Autodesk Inventor part; units mm, degrees
ref_plane "YZ Plane" through (0, 0, 0) normal (1, 0, 0) x (0, 1, 0)
ref_plane "XZ Plane" through (0, 0, 0) normal (0, 1, 0) x (-1, 0, 0)
ref_plane "XY Plane" through (0, 0, 0) normal (0, 0, 1) x (1, 0, 0)
sketch "Sketch1" plane through (0, 0, 0) normal (1, 0, 0) x (0, 1, 0)
  circle A0 centre (0, 0) radius 57.5
  line L0 (0, 0) -> (22.0043, 53.1231)
  line L1 (0, 0) -> (22.0043, -53.1231)
  line L2 (22.0043, 53.1231) -> (22.0043, -53.1231) construction
  line L3 (22.0043, 53.1231) -> (24.3004, 58.6664)
  line L4 (22.0043, -53.1231) -> (24.3004, -58.6664)
  circle A1 centre (0, 0) radius 63.5
  line L5 (22.0043, -53.1231) -> (207.792, -211.7609)
  line L6 (0, 0) -> (0, -50)
  line L7 (94.6424, 43.3552) -> (292.208, -112.8976)
  line L8 (92.474, 38.6955) -> (288.9589, -116.7027)
  line L9 (26.9658, -50.7848) -> (211.0388, -207.9584)
  line L10 (292.208, -112.8976) -> (207.792, -211.7609)
  circle A2 centre (250, -162.3292) radius 10
  circle A3 centre (250, -162.3292) radius 76
  line L11 (94.6424, 43.3552) -> (27.9796, 57.0034)
  line L12 (22.0043, 53.1231) -> (92.474, 38.6955)
  line L13 (0, 0) -> (0, -77.5)
  point P0 (22.0043, 0)
  point P1 (250.5574, -86.3313)
  point P2 (259.3441, -86.9058)
  point P3 (177.842, -186.1875)
  point P4 (175.5639, -177.6676)
  point P5 (243.5065, -169.9341)
  point P6 (256.4935, -154.7244)
  point P7 (27.0643, -57.4436)
  point P8 (39.7995, 49.4798)
  point P9 (31.8357, -54.943)
  dimension "d0" = 115
  dimension "d1" = 135
  dimension "d2" = 6
  dimension "d6" = 5
  dimension "d7" = 5
  dimension "d8" = 90
  dimension "d9" = 130
  dimension "d11" = 50
  dimension "d14" = 20
  dimension "d16" = 152
  dimension "d17" = 250
  dimension "d18" = 5
  dimension "d24" = 77.5
  dimension "d26" = 264
extrude "Extrusion1" add sketch "Sketch1" against normal blind 280 contours L3 A1 L12 | L9 A1 L5 A0 | A1 L11 L7 A3 L8 L12 | L9 A3 L5 A1
extrude "Extrusion2" add sketch "Sketch1" along normal blind 5 contours A0 L12 A1 L9 | L3 A1 L12 | L9 A1 L5 A0 | L12 L8 A3 L9 A1 | A1 L11 L7 A3 L8 L12 | L9 A3 L5 A1
ref_plane "Work Plane1" through (-140, 0, 0) normal (-1, 0, 0) x (0, 0, 1)
mirror "Mirror1" about plane through (-140, 0, 0) normal (-1, 0, 0) of "Extrusion2"
sketch "Sketch2" plane through (5, 0, 0) normal (1, 0, 0) x (0, 0, -1)
  line L0 (86.9058, 259.3441) -> (-43.3552, 94.6424)
  line L1 (-43.3552, 94.6424) -> (-57.0034, 27.9796)
  arc A0 (-57.0034, 27.9796) -> (-58.6664, 24.3004) centre (0, 0) ccw
  line L2 (-58.6664, 24.3004) -> (-53.1231, 22.0043)
  arc A1 (53.1231, 22.0043) -> (-53.1231, 22.0043) centre (0, 0) ccw
  line L3 (53.1231, 22.0043) -> (186.1875, 177.842)
  arc A2 (86.9058, 259.3441) -> (186.1875, 177.842) centre (162.3292, 250) ccw
  circle A3 centre (0, 0) radius 63.5
  circle A4 centre (-21.0494, 66.7602) radius 1.65
  line L4 (-21.0494, 66.7602) -> (0, 0) construction
  line L5 (0, 0) -> (21.0494, 66.7602) construction
  line L6 (-21.0494, 66.7602) -> (21.0494, 66.7602) construction
  circle A5 centre (21.0494, 66.7602) radius 1.65
  point P0 (0, 66.7602)
  dimension "d19" = 3.3
  dimension "d20" = 70
  dimension "d21" = 35
extrude "Extrusion3" cut sketch "Sketch2" against normal through all contours A4 | A5
ref_plane "Work Plane2" through (0, 259.3441, -86.9058) normal (0, 0.7729, -0.6345) x (1, 0, 0)
sketch "Sketch3" plane through (0, 259.3441, -86.9058) normal (0, 0.7729, -0.6345) x (1, 0, 0)
  line L0 (-314.1788, 142.1673) -> (47.7858, 142.1673)
  line L1 (47.7858, 142.1673) -> (47.7858, -28.3874)
  line L2 (47.7858, -28.3874) -> (-314.1788, -28.3874)
  line L3 (-314.1788, -28.3874) -> (-314.1788, 142.1673)
  point P0 (0, 97.3835)
extrude "Extrusion4" cut sketch "Sketch3" against normal blind 3
properties part number "CANALETA_GUIA" material "Steel, Mild, Welded"
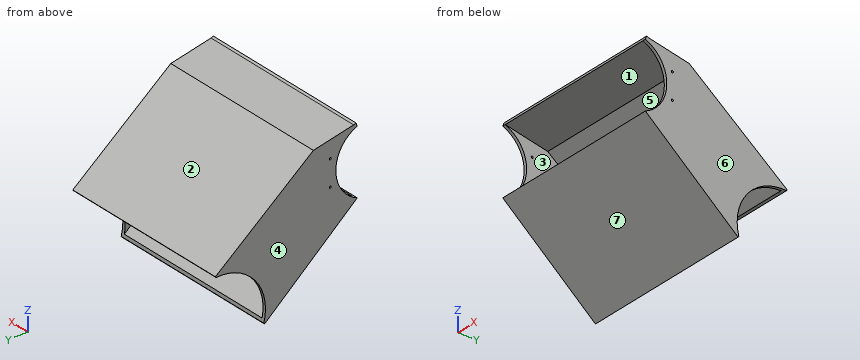
For this review, take the finished solid that the model builds, in its own axes (mm). Face numbers are marked on the shaded views. A direction names the side the tool comes from. Give positions to 0.01 mm unless a question says otherwise; leave off trailing zeros. Loops run counter-clockwise (first coordinate to the right, second up) from the corner with the lowest first, then second, coordinate; pieces in that order, holes last. Notation, with made-up numbers: M -31,0.25 L 23,0.25 A21 cw 23,17.25 Z; hole C 71.5,64 d9. An arc over 180 degrees is marked long. One line per item, written item: value. Start each with the question number.
Q1. Add section A-A (x = -240.5). Give the boundary of the cut face in (y, z), and give its area (3 significant figures).
Q2. Clearance check with flat-ended pins moving along their axes: pin 1 Ø2 at (x, z) = (-91.5, -36) entering from -Y; pin 2 Ø2.5 at (y, z) = (66.76, 21.05) entering from +X; pin 3 Ø3 at (x, y) = (-237.5, 105.5) entering from +Z; pin 4 Ø4 at (x, z) = (-157.5, -93.5) entering from +Y. State where each tip first meets the part, or that it passes through.
Q3. Machinability: for the marked faces 1, 2 and 3, which of the approach directions +Z, -Z, +X, -X, +Y, -Y give a long, thin tool a straight path to every point of the face, cutting with its end or side? Answer none if there is none.
Q4. Draft analysis for pull direction X (two halves, no side actions). For the marked faces 4, 5, 6 and 7, state which applies: released by +X, released by -X, zero draft, split by the parting line, or undercut.
Q5. Add section D-D (y = 53). Give the boundary of the cut face in (x, z).
Q6. Add section C-C (z = -78.5). Give the boundary of the cut face in (x, y), and give its area (3 significant figures).
Q7. For L1, parallel to X at y = 129, z = -44; L2, parallel to Z at x = -35.5, y = 49.5; L3, parallel to Z at x = -135, y = 169, list the stretches that pass through material, from the lowest coordinate up.
Q8. Add section B-B (y = 155.5). Give the boundary of the cut face in (x, z).
Reply:
1. outline: M 22,-53.12 L 175.56,-184.24 L 176.79,-182.73 A76 cw 175.56,-177.67 L 26.97,-50.78 A57.5 cw Z; M 22,53.12 L 92.47,38.7 L 250.56,-86.33 A76 cw 255.75,-86.55 L 256.99,-85.04 L 94.64,43.36 L 27.98,57 A63.5 ccw 24.3,58.67 Z
1. area: 2,380 mm²
2. pin 1: y = 185.65
2. pin 2: through
2. pin 3: z = 35.95
2. pin 4: y = 79.33
3. face 1: -Y
3. face 2: +Z, +X, -X, +Y
3. face 3: none
4. face 4: released by -X
4. face 5: undercut
4. face 6: released by +X
4. face 7: zero draft
5. outline: M -285,-79.59 L 5,-79.59 L 5,-22.3 L 0,-22.3 L 0,-73.01 L -280,-73.01 L -280,-22.3 L -285,-22.3 Z; M -285,22.3 L -280,22.3 L -280,46.78 L 0,46.78 L 0,22.3 L 5,22.3 L 5,51.88 L -285,51.88 Z
6. outline: M -285,51.72 L 5,51.72 L 5,248.72 L -285,248.72 Z; hole M -280,59.42 L 0,59.42 L 0,240.66 L -280,240.66 Z
6. area: 6,380 mm²
7. L1: -285 to -280, 0 to 5
7. L2: -76.6 to -70.03, 47.49 to 52.6
7. L3: -178.64 to -172.06, -21.83 to -15.45
8. outline: M -285,-167.11 L 5,-167.11 L 5,-4.78 L -285,-4.78 Z; hole M -280,-160.54 L 0,-160.54 L 0,-11.15 L -280,-11.15 Z
